Can you work these out from the model? Positions are in its coordinate system, mm. Face numbers are marked on the shaded views. Coordinates: 2 decimals unless noted, no trailing zeros. Order: outer loops, then holes, each group sorted by start corner. A loop starts at its lowest first (then second) coordinate and runs counter-clockwise, first axis right, second up. Notation, with made-up numbers: (24, 13) - (67, 13) arc R35 ccw to (67, 52) - close; hole circle Ø9 at (70, 2). An arc over 180 degrees is marked (long way). Return JSON: item names as keys, results as strings. Group by question number.
1) Imagine slicing it at B-B (x = 14). Write out the boundary of the cut face in (y, z).
2) Imagine slicing it at A-A (y = 1.3). Write out the boundary of the cut face in (x, z).
3) If I drill on line 1 along X through (y, z) = (2.15, 21.5); line 2 along Z through (x, y) = (-17, 1.1); line 3 along Y through (x, z) = (16.5, -14.5), over which ranges is the centre line in solid material (lowest first)?
4) For pin 1 Ø8 at (x, z) = (-11.5, 19) entering from -Y, with a flat end and sliding along its axis, tell me the tip position at first contact or that it passes through.
5) Imagine slicing it at C-C (z = 0). Write out the boundary of the cut face in (x, y).
6) Imagine slicing it at D-D (x = 0). Write out the boundary of the cut face in (y, z), and give its area (3 significant figures).
7) If we mould it in two halves opening along Y, with no side actions, what happens to the marked faces 1 and 2? For each: pulls with the +Y half, pulls with the -Y half, needs draft (parallel to the pull), parting line crosses it, or undercut.
```python
from build123d import *

# Parameters (mm, degrees)
EXTRUDE_1_DEPTH = 3
SKETCH_2_R      = 17.5
EXTRUDE_2_DEPTH = 3


with BuildPart() as part:
    # 草图1 → 凸台-拉伸1 (new body)
    with BuildSketch(Plane(origin=(0, 0, 0), x_dir=(1, 0, 0), z_dir=(0, 1, 0))):
        with BuildLine():
            Line((16, -29.5), (-16, -29.5))
            ThreePointArc((-16, -29.5), (-19.535533906, -28.035533906), (-21, -24.5))
            Line((-21, -24.5), (-21, 24.5))
            ThreePointArc((-21, 24.5), (-19.535533906, 28.035533906), (-16, 29.5))
            Line((-16, 29.5), (16, 29.5))
            ThreePointArc((16, 29.5), (19.535533906, 28.035533906), (21, 24.5))
            Line((21, 24.5), (21, -24.5))
            ThreePointArc((21, -24.5), (19.535533906, -28.035533906), (16, -29.5))
        make_face()
        with BuildLine():
            Line((-11.5, 24.3), (-11.5, 20.7))
            ThreePointArc((-11.5, 20.7), (-14.5, 17.7), (-17.5, 20.7))
            Line((-17.5, 20.7), (-17.5, 24.3))
            ThreePointArc((-17.5, 24.3), (-14.5, 27.3), (-11.5, 24.3))
        make_face(mode=Mode.SUBTRACT)
        with BuildLine():
            Line((11.5, 24.3), (11.5, 20.7))
            ThreePointArc((11.5, 20.7), (14.5, 17.7), (17.5, 20.7))
            Line((17.5, 20.7), (17.5, 24.3))
            ThreePointArc((17.5, 24.3), (14.5, 27.3), (11.5, 24.3))
        make_face(mode=Mode.SUBTRACT)
        with BuildLine():
            Line((-11.5, -24.3), (-11.5, -20.7))
            ThreePointArc((-11.5, -20.7), (-14.5, -17.7), (-17.5, -20.7))
            Line((-17.5, -20.7), (-17.5, -24.3))
            ThreePointArc((-17.5, -24.3), (-14.5, -27.3), (-11.5, -24.3))
        make_face(mode=Mode.SUBTRACT)
        with BuildLine():
            Line((11.5, -24.3), (11.5, -20.7))
            ThreePointArc((11.5, -20.7), (14.5, -17.7), (17.5, -20.7))
            Line((17.5, -20.7), (17.5, -24.3))
            ThreePointArc((17.5, -24.3), (14.5, -27.3), (11.5, -24.3))
        make_face(mode=Mode.SUBTRACT)
    extrude(amount=EXTRUDE_1_DEPTH)

    # 草图2 → 凸台-拉伸2 (add)
    with BuildSketch(Plane.XZ):
        with Locations(Location((0, 0, 0), (0, 0, 90))):
            Circle(SKETCH_2_R)
    extrude(amount=EXTRUDE_2_DEPTH)


solid = part.part
```
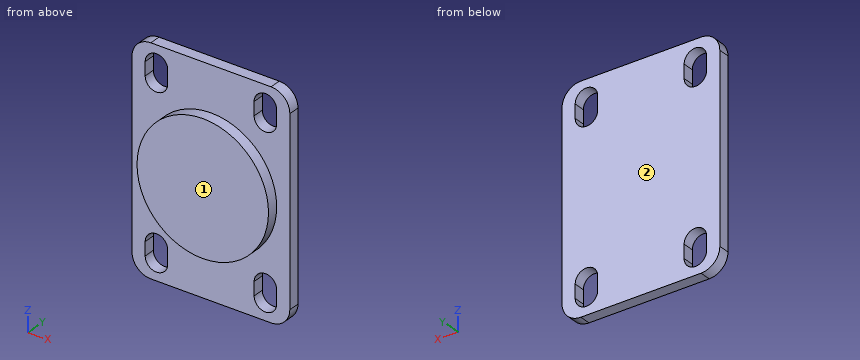
Calculated:
{
 "1": {"outline": "(-3, -10.5) - (0, -10.5) - (0, -17.74) - (3, -17.74) - (3, 17.74) - (0, 17.74) - (0, 10.5) - (-3, 10.5) - close; (0, -29.5) - (3, -29.5) - (3, -27.26) - (0, -27.26) - close; (0, 27.26) - (3, 27.26) - (3, 29.5) - (0, 29.5) - close"},
 "2": {"outline": "(-21, -24.5) arc R5 ccw to (-16, -29.5) - (16, -29.5) arc R5 ccw to (21, -24.5) - (21, 24.5) arc R5 ccw to (16, 29.5) - (-16, 29.5) arc R5 ccw to (-21, 24.5) - close; hole (-17.5, -24.3) arc R3 ccw to (-11.5, -24.3) - (-11.5, -20.7) arc R3 ccw to (-17.5, -20.7) - close; hole (-17.5, 20.7) arc R3 ccw to (-11.5, 20.7) - (-11.5, 24.3) arc R3 ccw to (-17.5, 24.3) - close; hole (11.5, -24.3) arc R3 ccw to (17.5, -24.3) - (17.5, -20.7) arc R3 ccw to (11.5, -20.7) - close; hole (11.5, 20.7) arc R3 ccw to (17.5, 20.7) - (17.5, 24.3) arc R3 ccw to (11.5, 24.3) - close"},
 "3": {"line 1": "-21 to -17.5, -11.5 to 11.5, 17.5 to 21", "line 2": "-29.4 to -25.96, -19.04 to 19.04, 25.96 to 29.4", "line 3": "0 to 3"},
 "4": {"pin 1": "y = 0"},
 "5": {"outline": "(-21, 0) - (-17.5, 0) - (-17.5, -3) - (17.5, -3) - (17.5, 0) - (21, 0) - (21, 3) - (-21, 3) - close"},
 "6": {"outline": "(-3, -17.5) - (0, -17.5) - (0, -29.5) - (3, -29.5) - (3, 29.5) - (0, 29.5) - (0, 17.5) - (-3, 17.5) - close", "area": "282 mm2"},
 "7": {"face 1": "pulls with the -Y half", "face 2": "pulls with the +Y half"}
}
